Work out the finished part from the listing and answer in its coordinate system (mm). A direction names the side the tool comes from. Round coordinates to 2 decimals unless told otherwise and drop trailing zeros. Loops run counter-clockwise (first coordinate to the right, second up) from the corner with the lowest first, then second, coordinate; pieces in that order, holes last.
from build123d import *

# Parameters (mm, degrees)
BOSS_EXTRUDE1_DEPTH      = 8
BOSS_EXTRUDE1_DEPTH_BACK = 8
BOSS_EXTRUDE2_DEPTH      = 4
BOSS_EXTRUDE2_DEPTH_BACK = 16
SKETCH2_R                = 8
SKETCH2_R_2              = 3.75
SKETCH2_2_R              = 3.75
CUT_EXTRUDE1_DEPTH       = 16


with BuildPart() as part:
    # Sketch1 → Boss-Extrude1 (new, two sides: drawn at the far end of the back side and taken through both)
    with BuildSketch(Plane.XY.offset(-BOSS_EXTRUDE1_DEPTH_BACK)):
        Polygon((-82, 0), (82, 0), (82, 12), (66, 12), (65.090074414, 14.5), (63.090074414, 14.5), (62.180148829, 12), (60, 12), (59.090074414, 14.5), (57.090074414, 14.5), (56.180148829, 12), (54, 12), (53.090074414, 14.5), (51.090074414, 14.5), (50.180148829, 12), (48, 12), (47.090074414, 14.5), (45.090074414, 14.5), (44.180148829, 12), (42, 12), (41.090074414, 14.5), (39.090074414, 14.5), (38.180148829, 12), (36, 12), (35.090074414, 14.5), (33.090074414, 14.5), (32.180148829, 12), (30, 12), (29.090074414, 14.5), (27.090074414, 14.5), (26.180148829, 12), (24, 12), (23.090074414, 14.5), (21.090074414, 14.5), (20.180148829, 12), (18, 12), (17.090074414, 14.5), (15.090074414, 14.5), (14.180148829, 12), (12, 12), (11.090074414, 14.5), (9.090074414, 14.5), (8.180148829, 12), (6, 12), (5.090074414, 14.5), (3.090074414, 14.5), (2.180148829, 12), (0, 12), (-0.909925586, 14.5), (-2.909925586, 14.5), (-3.819851171, 12), (-6, 12), (-6.909925586, 14.5), (-8.909925586, 14.5), (-9.819851171, 12), (-12, 12), (-12.909925586, 14.5), (-14.909925586, 14.5), (-15.819851171, 12), (-18, 12), (-18.909925586, 14.5), (-20.909925586, 14.5), (-21.819851171, 12), (-24, 12), (-24.909925586, 14.5), (-26.909925586, 14.5), (-27.819851171, 12), (-30, 12), (-30.909925586, 14.5), (-32.909925586, 14.5), (-33.819851171, 12), (-36, 12), (-36.909925586, 14.5), (-38.909925586, 14.5), (-39.819851171, 12), (-42, 12), (-42.909925586, 14.5), (-44.909925586, 14.5), (-45.819851171, 12), (-48, 12), (-48.909925586, 14.5), (-50.909925586, 14.5), (-51.819851171, 12), (-54, 12), (-54.909925586, 14.5), (-56.909925586, 14.5), (-57.819851171, 12), (-60, 12), (-60.909925586, 14.5), (-62.909925586, 14.5), (-63.819851171, 12), (-82, 12), align=None)
    extrude(amount=BOSS_EXTRUDE1_DEPTH + BOSS_EXTRUDE1_DEPTH_BACK)

    # Sketch2 → Boss-Extrude2 (add, two sides: drawn at the far end of the back side and taken through both)
    # profile 1 of 2: a face of its own
    with BuildSketch(Plane(origin=(0, 12, 0), x_dir=(1, 0, 0), z_dir=(0, 1, 0)).offset(-BOSS_EXTRUDE2_DEPTH_BACK)):
        with Locations(Location((82, 0, 0), (0, 0, 180))):
            Circle(SKETCH2_R)
        with Locations(Location((82, 0, 0), (0, 0, 180))):
            Circle(SKETCH2_R_2, mode=Mode.SUBTRACT)
    # profile 2 of 2: a face of its own
    with BuildSketch(Plane(origin=(0, 12, 0), x_dir=(1, 0, 0), z_dir=(0, 1, 0)).offset(-BOSS_EXTRUDE2_DEPTH_BACK)):
        with Locations((-82, 0)):
            Circle(SKETCH2_R)
        with Locations((-82, 0)):
            Circle(SKETCH2_R_2, mode=Mode.SUBTRACT)
    extrude(amount=BOSS_EXTRUDE2_DEPTH + BOSS_EXTRUDE2_DEPTH_BACK)

    # Sketch2_2 → Cut-Extrude1 (cut)
    with BuildSketch(Plane(origin=(0, 12, 0), x_dir=(1, 0, 0), z_dir=(0, 1, 0))):
        with Locations((-82, 0)):
            Circle(SKETCH2_2_R)
        with BuildLine():
            Line((82, -3.75), (82, 3.75))
            ThreePointArc((82, 3.75), (78.25, 0), (82, -3.75))
        make_face()
        with BuildLine():
            ThreePointArc((85.75, 0), (84.651650429, 2.651650429), (82, 3.75))
            Line((82, 3.75), (82, -3.75))
            ThreePointArc((82, -3.75), (84.651650429, -2.651650429), (85.75, 0))
        make_face()
    extrude(amount=-CUT_EXTRUDE1_DEPTH, mode=Mode.SUBTRACT)


solid = part.part
Item 1: Section A-A, the plane y = -2.5 is taken. Give the vertices of the cut face in (x, z), plus the area to 3 significant figures.
Item 2: Section D-D, the plane z = 1.75 is taken. State how many separate pieces and enclosed holes the cut face has, plus the area to 3 significant figures.
Item 3: For faces 1 (the face through (-90, 6, 0)), 2 (the face through (78.56, -4, 1.89)), determine the directions among +Z, -Z, +X, -X, +Y, -Y from which every point of the face is accessible in a straight line to the end or side of a thin tool.
Item 4: Determine the mould class of faces 3 (the face through (71, 12, 0)), 4 (the face through (-1, 7, 8)) for opening direction X: pulls with the +X half, pulls with the -X half, needs draft (parallel to the pull), parting line crosses it, or undercut.
Item 5: Section B-B, the plane y = 7.25 is taken. Give the vertices of the cut face in (x, z).
Item 6: Section C-C, the plane x = 68 is taken. Give the vertices of the cut face in (y, z).
Item 7: Each of these flat-tipped pins is pushed along its axis until it touches: P1, Ø5, axis at y = 12.5, z = 3.5, coming from the -X side; P2, Ø0.6, axis at x = 10, z = 1, coming from the +Y side; P3, Ø1.1, axis at x = -53, z = -3.5, coming from the +Y side; P4, Ø1, axis at x = 48.5, y = -1, coming from the -Z side. Where does it stop, or does it pass through?
Item 8: Straight lines are drawn through the part: line 1 (Z direction, x = -82, y = 13.15); line 2 (X direction, y = 7.5, z = 2.25); line 3 (Y direction, x = -58, z = -0.75). For each, find the intervals that lie inside material, in ascending order.
Answer below:
1. outline: circle Ø16 at (-82, 0); circle Ø16 at (82, 0); hole circle Ø7.5 at (-82, 0); hole circle Ø7.5 at (82, 0)
1. area: 314 mm2
2. separate pieces: 3
2. enclosed holes: 0
2. area: 2,300 mm2
3. face 1: none
3. face 2: +Z, -Z, +X, -X, -Y
4. face 3: undercut
4. face 4: needs draft
5. outline: (-82, -8) - (82, -8) arc R8 ccw to (82, 8) - (-82, 8) arc R8 ccw to start; hole circle Ø7.5 at (-82, 0); hole circle Ø7.5 at (82, 0)
6. outline: (0, -8) - (12, -8) - (12, 8) - (0, 8) - close
7. P1: stops at x = -89.94
7. P2: stops at y = 14.5
7. P3: stops at y = 12
7. P4: passes through
8. line 1: z = -8 to -3.75, 3.75 to 8
8. line 2: x = -89.68 to -85, -79 to 79, 85 to 89.68
8. line 3: y = 0 to 12
